from build123d import *

# Parameters (mm, degrees)
SKETCH1_R           = 2.1
BOSS_EXTRUDE1_DEPTH = 6.35
SKETCH2_R           = 2.1
CUT_EXTRUDE1_DEPTH  = 7.35
SKETCH3_R           = 2
CUT_EXTRUDE2_DEPTH  = 8


with BuildPart() as part:
    # Sketch1 → Boss-Extrude1 (new body)
    with BuildSketch(Plane.XY):
        Polygon((90, 6.35), (110, 6.35), (110, -29), (57.914505889, -29), (57.914505889, 0), (90, 0), align=None)
        with Locations((95.5, 3.175)):
            Circle(SKETCH1_R, mode=Mode.SUBTRACT)
        with Locations((104.5, 3.175)):
            Circle(SKETCH1_R, mode=Mode.SUBTRACT)
    extrude(amount=BOSS_EXTRUDE1_DEPTH)

    # Sketch2 → Cut-Extrude1 (cut, through all)
    with BuildSketch(Plane.XY.offset(6.35)):
        with Locations((70.935879417, -22.5)):
            Circle(SKETCH2_R)
        with Locations((83.957252945, -22.5)):
            Circle(SKETCH2_R)
        with Locations((96.978626472, -22.5)):
            Circle(SKETCH2_R)
        with Locations((93, -6)):
            Circle(SKETCH2_R)
        with Locations((77, -6)):
            Circle(SKETCH2_R)
    extrude(amount=-CUT_EXTRUDE1_DEPTH, mode=Mode.SUBTRACT)

    # Sketch3 → Cut-Extrude2 (cut)
    with BuildSketch(Plane(origin=(0, 0, 0), x_dir=(-1, 0, 0), z_dir=(0, 1, 0))):
        with Locations((-84, 3.175)):
            Circle(SKETCH3_R)
        with Locations((-63.914505889, 3.175)):
            Circle(SKETCH3_R)
    extrude(amount=-CUT_EXTRUDE2_DEPTH, mode=Mode.SUBTRACT)


solid = part.part
CAD build for the part. Positions are in the model's coordinates, mm. A direction names the side the tool comes from. Round coordinates to 2 decimals unless told otherwise and drop trailing zeros. Write each loop counter-clockwise with the first axis right and the second up, starting at its lowest first coordinate (ties: lowest second). Pieces come first, ordered by that corner, then holes. Notation, with made-up numbers: (33, 0) -> (75, 0) arc R25 cw to (75, 36) -> close; hole circle Ø5 at (-23.75, 33.5). An arc over 180 degrees is marked (long way). Answer as a JSON object with one key per item and string values.
(1) Band-saw the part on C-C, the plane y = -6. Count the separate pieces of the cut face and the enclosed holes in it, then the cut area to 3 significant figures.
Reported:
{"separate pieces": "3", "enclosed holes": "2", "area": "252 mm^2"}
(2) Pin check, flat tips, straight feed: P1, Ø3, axis at y = 4.5, z = 2, coming from the -X side; P2, Ø2, axis at x = 64, z = 3.5, coming from the +Y side; P3, Ø1.9, axis at x = 74, z = 3, coming from the +Y side. Stop position of each tip, or through.
Reported:
{"P1": "stops at x = 90", "P2": "stops at y = -8", "P3": "stops at y = 0"}
(3) Probe probe 1 along X at (y, z) = (-23.5, 1.5); probe 2 along X at (y, z) = (-22, 3); probe 3 along X at (y, z) = (2, 1). List the from-to ranges inside material, lowest first. Write a range as [from, to].
Reported:
{"probe 1": "x = [57.91, 69.09], [72.78, 82.11], [85.8, 95.13], [98.83, 110]", "probe 2": "x = [57.91, 68.9], [72.98, 81.92], [86, 94.94], [99.02, 110]", "probe 3": "x = [90, 93.76], [97.24, 102.76], [106.24, 110]"}
(4) Which spindle directions (+Z, -Z, +X, -X, +Y, -Y) get a long thin tool onto all of the face, cutting with end or side? Do faces 4 (the face through (85.96, -21.87, 3.22)), 5 (the face through (82.1, -3.9, 3.8)). Say none if no direction does.
Reported:
{"face 4": "+Z, -Z", "face 5": "+Y"}
(5) Two-plate mould, pull along Y, no slides. Class faces 1 (the face through (72.065, -20.729, 3.219)), 2 (the face through (84, -29, 3)), 3 (the face through (90, 3, 3)): +Y half, -Y half, draft (parallel to the pull), parting line (faces both ways), or undercut.
Reported:
{"face 1": "undercut", "face 2": "-Y half", "face 3": "draft"}
(6) Band-saw the part on B-B, the plane x = 104.5. List the corners of the cut face in (y, z) (3 decimals).
Reported:
{"outline": "(-29, 0) -> (1.075, 0) -> (1.075, 6.35) -> (-29, 6.35) -> close; (5.275, 0) -> (6.35, 0) -> (6.35, 6.35) -> (5.275, 6.35) -> close"}
(7) Band-saw the part on D-D, the plane x = 77. List the corners of the cut face in (y, z).
Reported:
{"outline": "(-29, 0) -> (-8.1, 0) -> (-8.1, 6.35) -> (-29, 6.35) -> close; (-3.9, 0) -> (0, 0) -> (0, 6.35) -> (-3.9, 6.35) -> close"}
(8) Band-saw the part on A-A, the plane y = -22.5. List the corners of the cut face in (x, z), then the cut area to 3 significant figures.
Reported:
{"outline": "(57.91, 0) -> (68.84, 0) -> (68.84, 6.35) -> (57.91, 6.35) -> close; (73.04, 0) -> (81.86, 0) -> (81.86, 6.35) -> (73.04, 6.35) -> close; (86.06, 0) -> (94.88, 0) -> (94.88, 6.35) -> (86.06, 6.35) -> close; (99.08, 0) -> (110, 0) -> (110, 6.35) -> (99.08, 6.35) -> close", "area": "251 mm^2"}
